The model under review builds one solid part; all positions refer to its coordinate system, in mm. Coordinates: 2 decimals unless noted, no trailing zeros. Order: outer loops, then holes, each group sorted by start corner. A loop starts at its lowest first (then second) coordinate and runs counter-clockwise, first axis right, second up. Notation, with made-up numbers: M 23.25,85 L 46.25,85 A23 cw 46.25,94 Z; hole C 8,56.25 d6. An arc over 180 degrees is marked long. Write each question's results on one line, items separated by ' | '.
Autodesk Inventor part; units mm, degrees
ref_plane "YZ Plane" through (0, 0, 0) normal (1, 0, 0) x (0, 1, 0)
ref_plane "XZ Plane" through (0, 0, 0) normal (0, 1, 0) x (-1, 0, 0)
ref_plane "XY Plane" through (0, 0, 0) normal (0, 0, 1) x (1, 0, 0)
sketch "Sketch6" plane through (0, 0, 0) normal (0, 1, 0) x (-1, 0, 0)
  line L0 (360, -990) -> (-360, -990)
  line L1 (-360, -990) -> (-360, 990)
  line L2 (-360, 990) -> (360, 990)
  line L3 (360, 990) -> (360, -990)
  line L4 (360, -990) -> (-360, 990) construction
  line L5 (-360, -990) -> (360, 990) construction
  point P0 (0, 0)
  dimension "d52" = 720
  dimension "d53" = 1980
extrude "Plate2" add sketch "Sketch6" along normal blind 0.5
sketch "Sketch11" plane through (-359.5, 0, 990) normal (-1, 0, 0) x (0, -1, 0)
  line L0 (0, -1980) -> (0, 0)
  line L1 (0, 0) -> (-10, 0)
  line L2 (-10, 0) -> (-10, -1980)
  line L3 (-10, -1980) -> (0, -1980)
edge flange "Flange2" height 10 angle 90 thickness 0.5 bend radius 0.5 thickness toward (-1, 0, 0) relief tear relief width 0.5 relief depth 0.25 edges at (-360, 0.5, 0) wall of the first edge with corners at (-359.5, 0, -990) (-359.5, 0, 990) (-359.5, 10, 990) (-359.5, 10, -990)
bend "Bend3"
corner "Corner3"
sketch "Sketch12" plane through (-360, 9.5, 990) normal (0, 1, 0) x (-1, 0, 0)
  line L0 (0, -1980) -> (0, 0)
  line L1 (0, 0) -> (-10, 0)
  line L2 (-10, 0) -> (-10, -1980)
  line L3 (-10, -1980) -> (0, -1980)
edge flange "Flange3" height 10 angle 90 thickness 0.5 bend radius 0.5 thickness toward (0, 1, 0) relief tear relief width 0.5 relief depth 0.25 edges at (-359.5, 10, 0) wall of the first edge with corners at (-360, 9.5, -990) (-360, 9.5, 990) (-350, 9.5, 990) (-350, 9.5, -990)
bend "Bend4"
corner "Corner4"
sketch "Sketch13" plane through (359.5, 0, -990) normal (1, 0, 0) x (0, 1, 0)
  line L0 (0, 1980) -> (0, 0)
  line L1 (0, 0) -> (10, 0)
  line L2 (10, 0) -> (10, 1980)
  line L3 (10, 1980) -> (0, 1980)
edge flange "Flange4" height 10 angle 90 thickness 0.5 bend radius 0.5 thickness toward (1, 0, 0) relief tear relief width 0.5 relief depth 0.25 edges at (360, 0.5, 0) wall of the first edge with corners at (359.5, 0, 990) (359.5, 0, -990) (359.5, 10, -990) (359.5, 10, 990)
bend "Bend5"
corner "Corner5"
sketch "Sketch14" plane through (360, 9.5, -990) normal (0, 1, 0) x (-1, 0, 0)
  line L0 (0, 1980) -> (0, 0)
  line L1 (0, 0) -> (10, 0)
  line L2 (10, 0) -> (10, 1980)
  line L3 (10, 1980) -> (0, 1980)
edge flange "Flange5" height 10 angle 90 thickness 0.5 bend radius 0.5 thickness toward (0, 1, 0) relief tear relief width 0.5 relief depth 0.25 edges at (359.5, 10, 0) wall of the first edge with corners at (360, 9.5, 990) (360, 9.5, -990) (350, 9.5, -990) (350, 9.5, 990)
bend "Bend6"
corner "Corner6"
equation "\"d53\" = ЖАБРЫ_базовая_длина_дл_лист"
equation "\"d54\" = Thickness"
equation "\"d84\" = BendReliefWidth"
equation "\"d85\" = BendReliefDepth"
equation "\"d86\" = MinimumRemnant"
equation "\"d87\" = TransitionRadius"
equation "\"d90\" = BendRadius"
equation "\"d91\" = CornerReliefSize"
equation "\"d92\" = GapSize"
equation "\"d93\" = JacobiRadiusSize"
equation "\"d94\" = BendReliefWidth"
equation "\"d95\" = BendReliefDepth"
equation "\"d96\" = MinimumRemnant"
equation "\"d97\" = TransitionRadius"
equation "\"d100\" = BendRadius"
equation "\"d101\" = CornerReliefSize"
equation "\"d102\" = GapSize"
equation "\"d103\" = JacobiRadiusSize"
equation "\"d104\" = BendReliefWidth"
equation "\"d105\" = BendReliefDepth"
equation "\"d106\" = MinimumRemnant"
equation "\"d107\" = TransitionRadius"
equation "\"d110\" = BendRadius"
equation "\"d111\" = CornerReliefSize"
equation "\"d112\" = GapSize"
equation "\"d113\" = JacobiRadiusSize"
equation "\"d114\" = BendReliefWidth"
equation "\"d115\" = BendReliefDepth"
equation "\"d116\" = MinimumRemnant"
equation "\"d117\" = TransitionRadius"
equation "\"d120\" = BendRadius"
equation "\"d121\" = CornerReliefSize"
equation "\"d122\" = GapSize"
equation "\"d123\" = JacobiRadiusSize"
equation "\"BendRadius\" = Thickness"
equation "\"BendReliefWidth\" = Thickness"
equation "\"BendReliefDepth\" = 0.5 * Thickness"
equation "\"CornerReliefSize\" = 4 * Thickness"
equation "\"MinimumRemnant\" = 2 * Thickness"
equation "\"TransitionRadius\" = BendRadius"
equation "\"JacobiRadiusSize\" = BendRadius"
equation "\"GapSize\" = Thickness"
properties part number "MSC 806 sheet gills" material "Stainless Steel"
1) To check wall thickness, follow line 1 along X through (y, z) = (3, -92); line 2 along X through (y, z) = (0.75, -78); line 3 along Y through (x, z) = (195, 610.5). State the ranges of each line that lie inside material, in increasing order.
Solutions:
line 1: -360 to -359.5, 359.5 to 360 | line 2: -359.97 to -359.43, 359.43 to 359.97 | line 3: 0 to 0.5
2) Take a section at C-C on x = -114.5. State the section outline as (y, z) points, plus the area to 3 significant figures.
Solutions:
outline: M 0,-990 L 0.5,-990 L 0.5,990 L 0,990 Z | area: 990 mm2
3) Take a section at A-A on y = 6.25. State the section outline as (x, z) points, plus the area to 3 significant figures.
Solutions:
outline: M -360,-990 L -359.5,-990 L -359.5,990 L -360,990 Z; M 359.5,-990 L 360,-990 L 360,990 L 359.5,990 Z | area: 1,980 mm2
4) The part is to be moulded in two halves that separate along X. For faces 1 (the flat face through (5, 0.5, 14)), 2 (the flat face through (5, 0, 14)), say which applies: pulls with the +X half, pulls with the -X half, needs draft (parallel to the pull), parting line crosses it, or undercut.
Solutions:
face 1: undercut | face 2: needs draft
5) Take a section at B-B on z = 733.5. State the section outline as (x, y) points.
Solutions:
outline: M -360,1 A1 ccw -359,0 L 359,0 A1 ccw 360,1 L 360,9 A1 ccw 359,10 L 350,10 L 350,9.5 L 359,9.5 A0.5 cw 359.5,9 L 359.5,1 A0.5 cw 359,0.5 L -359,0.5 A0.5 cw -359.5,1 L -359.5,9 A0.5 cw -359,9.5 L -350,9.5 L -350,10 L -359,10 A1 ccw -360,9 Z
6) For pin 1 (8 mm diameter, centred on x = 10, z = 440, fed in from +Y), flat-tipped, find the tip position at first contact; note if it passes through.
Solutions:
pin 1: y = 0.5
